Autodesk Inventor part; units mm, degrees
ref_plane "YZ Plane" through (0, 0, 0) normal (1, 0, 0) x (0, 1, 0)
ref_plane "XZ Plane" through (0, 0, 0) normal (0, 1, 0) x (-1, 0, 0)
ref_plane "XY Plane" through (0, 0, 0) normal (0, 0, 1) x (1, 0, 0)
sketch "Sketch20" plane through (0, 0, 0) normal (0, 1, 0) x (-1, 0, 0)
  line L0 (57.5, -22.5) -> (-57.5, -22.5)
  line L1 (-57.5, -22.5) -> (-57.5, 22.5)
  line L2 (-57.5, 22.5) -> (57.5, 22.5)
  line L3 (57.5, 22.5) -> (57.5, -22.5)
  circle A0 centre (45, 0) radius 6
  circle A1 centre (-45, 0) radius 6
  point P0 (0, 0)
  dimension "d92" = 115
  dimension "d93" = 45
  dimension "d94" = 57.5
  dimension "d95" = 22.5
  dimension "d97" = 45
  dimension "d98" = 90
  dimension "d99" = 12
  dimension "d100" = 12
extrude "Extrusion17" add sketch "Sketch20" along normal blind 87
sketch "Sketch21" plane through (57.5, 0, -22.5) normal (0, 0, -1) x (-1, 0, 0)
  line L0 (115, 0) -> (115, 87)
  line L1 (0, 87) -> (115, 87)
  line L2 (0, 0) -> (0, 87)
  line L3 (57.5, 0) -> (57.5, 87) construction
  line L4 (115, 43.5) -> (0, 43.5) construction
  circle A0 centre (57.5, 43.5) radius 31.75
  dimension "d103" = 63.5
hole "Hole1" at (0, 43.5, -22.5) direction (0, 0, 1) diameter 63.5 end through all
equation "\"d100\" = d99"
properties part number "2.5 CIM mount" material "Polypropylene"
The model under review builds one solid part; all positions refer to its coordinate system, in mm. Coordinates: 2 decimals unless noted, no trailing zeros. Loops run counter-clockwise (first coordinate to the right, second up) from the corner with the lowest first, then second, coordinate; pieces in that order, holes last.
(1) Wall thickness on L1, parallel to Z at x = 45, y = 68; L2, parallel to X at y = 43.5, z = 11; L3, parallel to Y at x = 0, z = 1: over which ranges is each line inside the solid? List them lowest first.
Determined:
L1: z = -22.5 to -6, 6 to 22.5
L2: x = -57.5 to -31.75, 31.75 to 57.5
L3: y = 0 to 11.75, 75.25 to 87
(2) Consider section C-C, the plane z = 0. Give the boundary of the cut face in (x, y), plus the area to 3 significant figures.
Determined:
outline: (-57.5, 0) - (-51, 0) - (-51, 87) - (-57.5, 87) - close; (-39, 0) - (39, 0) - (39, 87) - (-39, 87) - close; (51, 0) - (57.5, 0) - (57.5, 87) - (51, 87) - close; hole circle Ø63.5 at (0, 43.5)
area: 4,750 mm2
(3) Consider section D-D, the plane z = 19.5. Give the boundary of the cut face in (x, y).
Determined:
outline: (-57.5, 0) - (57.5, 0) - (57.5, 87) - (-57.5, 87) - close; hole circle Ø63.5 at (0, 43.5)
(4) Consider section B-B, the plane y = 43.5. Give the boundary of the cut face in (x, z), plus the area to 3 significant figures.
Determined:
outline: (-57.5, -22.5) - (-31.75, -22.5) - (-31.75, 22.5) - (-57.5, 22.5) - close; (31.75, -22.5) - (57.5, -22.5) - (57.5, 22.5) - (31.75, 22.5) - close; hole circle Ø12 at (-45, 0); hole circle Ø12 at (45, 0)
area: 2,090 mm2
(5) Draft analysis for pull direction X (two halves, no side actions). For faces 1 (the flat face through (-57.5, 43, 0)), 2 (the flat face through (1, 87, 0)), 3 (the cylindrical face through (30.995, 36.617, 0.315)), state which applies: +X half, -X half, draft (parallel to the pull), parting line (faces both ways), or undercut.
Determined:
face 1: -X half
face 2: draft
face 3: undercut
(6) Consider section A-A, the plane x = 0. Give the boundary of the cut face in (y, z).
Determined:
outline: (0, -22.5) - (11.75, -22.5) - (11.75, 22.5) - (0, 22.5) - close; (75.25, -22.5) - (87, -22.5) - (87, 22.5) - (75.25, 22.5) - close
